Autodesk Fusion 360 part; units mm, degrees
sketch "Sketch1" plane through (0, 0, 0) normal (1, 0, 0) x (0, 1, 0)
  circle A0 centre (-25, 25) radius 2.975
  circle A1 centre (-25, 25) radius 5
  dimension "d1" = 5.95
  dimension "d4" = 10
extrude "Extrude1" add sketch "Sketch1" along normal blind 5 contours A0
extrude "Extrude2" add sketch "Sketch1" against normal blind 2 contours A0 | A1
chamfer "Chamfer1" distance 2 angle 45 1 edges at (-2, -29.6616, 26.8081) measured on face at (-2, -27.3344, 24.5087)
Work out the finished part from the listing and answer in its coordinate system (mm). A direction names the side the tool comes from. Give positions to 0.01 mm unless a question says otherwise; leave off trailing zeros. Order: outer loops, then holes, each group sorted by start corner. A loop starts at its lowest first (then second) coordinate and runs counter-clockwise, first axis right, second up.
1. Section C-C, the plane x = 0.75 is taken. Determine the outline of the cut face in (y, z) (3 decimals), and give its area (3 significant figures).
Result sheet:
outline: circle Ø5.95 at (-25, 25)
area: 27.8 mm2
2. For faces 1 (the cylindrical face through (2.465, -27.972, 24.869)), 2 (the flat face through (-2, -25, 25)), determine the directions among +Z, -Z, +X, -X, +Y, -Y from which every point of the face is accessible in a straight line to the end or side of a thin tool.
Result sheet:
face 1: +X
face 2: +Z, -Z, -X, +Y, -Y
3. Straight lines are drawn through the part: L1, parallel to X at y = -23.5, z = 28.5; L2, parallel to X at y = -28, z = 22; L3, parallel to Z at x = -1.25, y = -22. For each, find the intervals that lie inside material, in ascending order.
Result sheet:
L1: x = -1.19 to 0
L2: x = -0.76 to 0
L3: z = 22.75 to 27.25
4. Each of these flat-tipped pins is pushed along its axis until it touches: P1, Ø2, axis at x = 0, z = 26.5, coming from the +Y side; P2, Ø2, axis at x = 4, z = 24, coming from the -Y side (3 decimals); P3, Ø1, axis at x = -1, y = -27.5, coming from the -Z side. Where does it stop, or does it pass through?
Result sheet:
P1: stops at y = -20.03
P2: stops at y = -27.975
P3: stops at z = 21.18
